Autodesk Inventor part; units mm, degrees
ref_plane "YZ Plane" through (0, 0, 0) normal (1, 0, 0) x (0, 1, 0)
ref_plane "XZ Plane" through (0, 0, 0) normal (0, 1, 0) x (-1, 0, 0)
ref_plane "XY Plane" through (0, 0, 0) normal (0, 0, 1) x (1, 0, 0)
sketch "Sketch1" plane through (0, 0, 0) normal (1, 0, 0) x (0, 1, 0)
  line L0 (0, 0) -> (0, -9) construction
  line L1 (2, 0) -> (2, -9)
  line L2 (2, -9) -> (3, -9)
  line L3 (3, -9) -> (3, -7.5)
  line L4 (3, -7.5) -> (2.5, -7.5)
  line L5 (2.5, -7.5) -> (2.5, 0)
  line L6 (2.5, 0) -> (2, 0)
  line L7 (0, 0) -> (7.91, 0) construction
  dimension "d0" = 9
  dimension "d1" = 2
  dimension "d2" = 2.5
  dimension "d3" = 3
  dimension "d4" = 1.5
  dimension "d5" = 9
revolve "Revolution1" add sketch "Sketch1" angle 360 about axis through (0, 0, 0) along (0, 0, -1)
chamfer "Chamfer1" distance 0.15 angle 45 3 edges at (0, -3, -7.5) (0, -3, -9) (0, -2.5, 0)
properties part number "Component 5(Ram Bearing)"
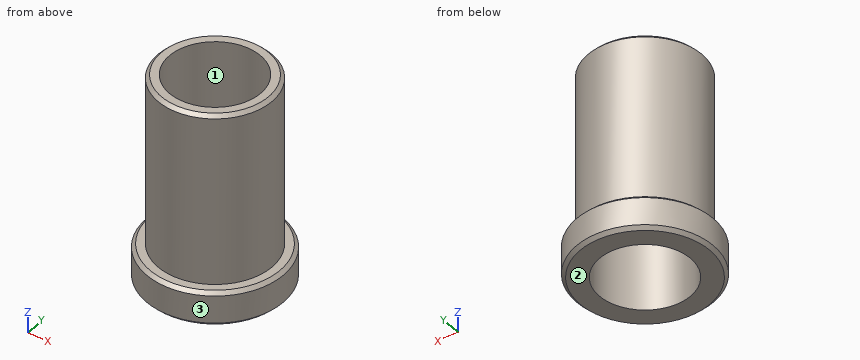
Read the model definition and answer for the solid it produces. Units are mm, in the model's axes. Face numbers are marked on the shaded views. Give positions to 0.01 mm unless a question says otherwise; leave off trailing zeros. Write each loop counter-clockwise with the first axis right and the second up, starting at its lowest first coordinate (ties: lowest second). Pieces come first, ordered by that corner, then holes. Notation, with made-up numbers: M 56.5,55.25 L 82.5,55.25 A29 ccw 82.5,94.25 Z; hole C 22,40.25 d5. An arc over 180 degrees is marked long. Put each result on its own line as item: value. Start each with the question number.
1. The part is cut by section C-C, the plane z = -4. Give the vertices of the cut face in (x, y).
2. For a pull along Y with two mould halves and no side action, classify the marked faces 1, 2 and 3 as released by +Y, released by -Y, zero draft, split by the parting line, or undercut.
3. Each of these flat-tipped pins is pushed along its axis until it touches: pin 1 Ø1.5 at (y, z) = (1.5, -5.5) entering from -X; pin 2 Ø1.5 at (y, z) = (-2, -5) entering from +X; pin 3 Ø3 at (y, z) = (1.5, -7.5) entering from +X; pin 4 Ø2.5 at (x, y) = (0, 0) entering from -Z. Where does it stop, or does it pass through?
4. The part is cut by section A-A, the plane y = 0. Give the vertices of the cut face in (x, z), and give its area (3 significant figures).
5. Consider line 1 along X through (y, z) = (0, -5.75); line 2 along Z through (x, y) = (1.6, 2.15); line 3 along X through (y, z) = (1.3, -2.25). Determine where each line is inside the solid, lowest interval first.
Final values:
1. outline: C 0,0 d5; hole C 0,0 d4
2. face 1: undercut
2. face 2: zero draft
2. face 3: split by the parting line
3. pin 1: stops at x = -2.38
3. pin 2: stops at x = 2.17
3. pin 3: stops at x = 3
3. pin 4: passes through
4. outline: M -3,-8.85 L -2.85,-9 L -2,-9 L -2,0 L -2.35,0 L -2.5,-0.15 L -2.5,-7.5 L -2.85,-7.5 L -3,-7.65 Z; M 2,-9 L 2.85,-9 L 3,-8.85 L 3,-7.65 L 2.85,-7.5 L 2.5,-7.5 L 2.5,-0.15 L 2.35,0 L 2,0 Z
4. area: 10.4 mm²
5. line 1: x = -2.5 to -2, 2 to 2.5
5. line 2: z = -9 to -7.5
5. line 3: x = -2.14 to -1.52, 1.52 to 2.14
